from build123d import *

# Parameters (mm, degrees)
BOSS_EXTRUDE1_DEPTH  = 2.54
SKETCH2_W            = 8.89
SKETCH2_H            = 13.97
CUT_EXTRUDE1_DEPTH   = 7.62
SKETCH3_R            = 3.683
CUT_EXTRUDE2_DEPTH   = 7.62
LPATTERN1_COUNT      = 2
LPATTERN1_PITCH      = 27.5
SKETCH4_R            = 3.048
CUT_EXTRUDE3_DEPTH   = 7.62
SKETCH6_W            = 6.35
SKETCH6_H            = 2.54
CUT_EXTRUDE5_DEPTH   = 2.54
FILLET1_R            = 1.27
LPATTERN4_COUNT      = 2
LPATTERN4_PITCH      = 228.6
LPATTERN4_COUNT_DIR2 = 2
LPATTERN4_PITCH_DIR2 = 50.8
LPATTERN5_COUNT      = 2
LPATTERN5_PITCH      = 75


with BuildPart() as part:
    # Sketch1 → Boss-Extrude1 (new body)
    with BuildSketch(Plane.XY):
        with BuildLine():
            Line((114.3, -31.75), (-114.3, -31.75))
            ThreePointArc((-114.3, -31.75), (-146.05, 0), (-114.3, 31.75))
            Line((-114.3, 31.75), (114.3, 31.75))
            ThreePointArc((114.3, 31.75), (146.05, 0), (114.3, -31.75))
        make_face()
    extrude(amount=BOSS_EXTRUDE1_DEPTH)

    # Sketch2 → Cut-Extrude1 (cut)
    with BuildSketch(Plane.XY.offset(2.54)):
        with Locations((-101.6, 0)):
            Rectangle(SKETCH2_W, SKETCH2_H)
    extrude(amount=-CUT_EXTRUDE1_DEPTH, mode=Mode.SUBTRACT)

    # Sketch3 → Cut-Extrude2 (cut)
    with BuildSketch(Plane.XY.offset(2.54)):
        with Locations((4.445, 0)):
            Circle(SKETCH3_R)
    cut_extrude2 = extrude(amount=-CUT_EXTRUDE2_DEPTH, mode=Mode.SUBTRACT)

    # LPattern1: Cut-Extrude2 ×2
    with Locations(*[(i * LPATTERN1_PITCH, 0, 0) for i in range(1, LPATTERN1_COUNT)]):
        add(cut_extrude2, mode=Mode.SUBTRACT)

    # Sketch4 → Cut-Extrude3 (cut)
    with BuildSketch(Plane.XY.offset(2.54)):
        with Locations((71.545, -0.635)):
            Circle(SKETCH4_R)
    extrude(amount=-CUT_EXTRUDE3_DEPTH, mode=Mode.SUBTRACT)

    # Sketch6 → Cut-Extrude5 (cut)
    with BuildSketch(Plane.XY.offset(2.54)):
        with Locations((55.289, -4.953)):
            Rectangle(SKETCH6_W, SKETCH6_H)
    cut_extrude5 = extrude(amount=-CUT_EXTRUDE5_DEPTH, mode=Mode.SUBTRACT)

    # Fillet1
    fillet1_edges = [part.edges().sort_by_distance(p)[0] for p in [
        (0, -31.75, 2.54),
        (-146.05, 0, 2.54),
        (0, 31.75, 2.54),
        (146.05, 0, 2.54),
        (146.05, 0, 0),
        (0, -31.75, 0),
        (-146.05, 0, 0),
        (0, 31.75, 0),
    ]]
    fillet(fillet1_edges, radius=FILLET1_R - 0.0001)  # a hair under: the kernel refuses the full size

    # Sketch9 → CSK for M5 Flat Head Machine Screw2 (revolve, cut)
    with BuildSketch(Plane(origin=(-114.3, 25.4, 2.54), x_dir=(0, -1, 0), z_dir=(1, 0, 0))):
        Polygon((0, 0), (0, 2.54), (2.75, 2.54), (2.75, 2.45), (5.2, 0), align=None)
    csk_for_m5_flat_head_machine_screw2 = revolve(axis=Axis((-114.3, 25.4, 8.89), (0, 0, -1)), mode=Mode.SUBTRACT)

    # LPattern4: CSK for M5 Flat Head Machine Screw2 2 × 2
    with Locations(*[(i * LPATTERN4_PITCH, -j * LPATTERN4_PITCH_DIR2, 0) for i in range(LPATTERN4_COUNT) for j in range(LPATTERN4_COUNT_DIR2) if (i, j) != (0, 0)]):
        add(csk_for_m5_flat_head_machine_screw2, mode=Mode.SUBTRACT)

    # LPattern5: Cut-Extrude5 ×2
    with Locations(*[(-i * LPATTERN5_PITCH, 0, 0) for i in range(1, LPATTERN5_COUNT)]):
        add(cut_extrude5, mode=Mode.SUBTRACT)


solid = part.part
Geometry: final body of the model. Coordinates: model frame, mm. Give positions to 0.01 mm unless a question says otherwise; leave off trailing zeros. Answer as a JSON object with one key per item and string values.
Q1. Section A-A (z = 0.7). State how many separate pieces and enclosed holes the cut face has, plus the area to 3 significant figures.
Entries:
{"separate pieces": "1", "enclosed holes": "10", "area": "17,200 mm^2"}
Q2. Material intervals for probe 1 along X at (y, z) = (-24, 1.45); probe 2 along Y at (x, z) = (-20.5, 1.5); probe 3 along Y at (x, z) = (0, 1.5), sorted ascending.
Entries:
{"probe 1": "x = -135.07 to -118.16, -110.44 to 110.44, 118.16 to 135.07", "probe 2": "y = -31.73 to -6.22, -3.68 to 31.73", "probe 3": "y = -31.73 to 31.73"}
Q3. First-contact query: pin 1 (5 mm diameter, centred on x = -114.3, y = 25.4, fed in from -Z); pin 2 (1 mm diameter, centred on x = -33, y = 13, fed in from -Z); pin 3 (1.3 mm diameter, centred on y = -1, z = 0.5, fed in from -X); pin 4 (1.3 mm diameter, centred on y = -0.5, z = 1, fed in from +X). Flat tips, straight axial feed; report the tip coordinate or a pass-through.
Entries:
{"pin 1": "passes through", "pin 2": "stops at z = 0", "pin 3": "stops at x = -146.03", "pin 4": "stops at x = 146.05"}
Q4. Draft query along Y for faces 1 (the conical face through (-116.748, 23.839, 0.243)), 2 (the flat face through (2, 7, 2.54)), 3 (the cylindrical face through (6.14, -3.27, 1.29)). Return one class per face: released by +Y, released by -Y, zero draft, split by the parting line, or undercut.
Entries:
{"face 1": "undercut", "face 2": "zero draft", "face 3": "undercut"}
